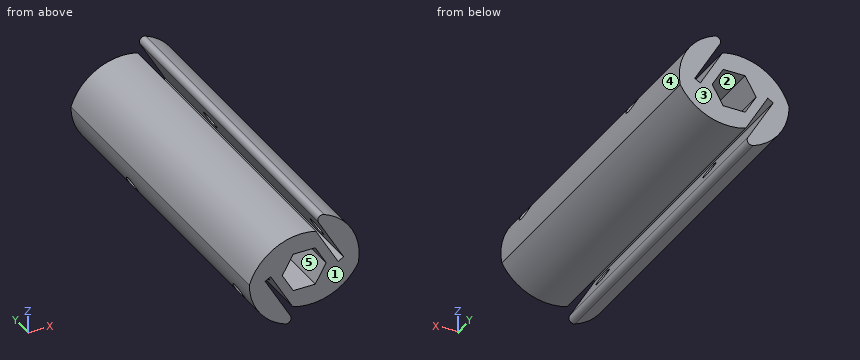
from build123d import *

# Parameters (mm, degrees)
BOSS_EXTRUDE1_DEPTH     = 114.3
CUT_EXTRUDE1_DEPTH      = 119.868393362
CUT_EXTRUDE1_DEPTH_BACK = 119.868393362
SKETCH2_R               = 3.175


with BuildPart() as part:
    # Sketch1 → Boss-Extrude1 (new body)
    with BuildSketch(Plane(origin=(0, 0, 0), x_dir=(1, 0, 0), z_dir=(0, 1, 0))):
        with BuildLine():
            Line((4.052973773, -12.538043503), (11.754987424, 0.80223546))
            Line((11.754987424, 0.80223546), (13.679728884, -0.30901454))
            Line((13.679728884, -0.30901454), (4.910037862, -15.498564956))
            ThreePointArc((4.910037862, -15.498564956), (5.078558502, -17.32430787), (6.856203481, -17.773434497))
            ThreePointArc((6.856203481, -17.773434497), (16.623747328, -9.303414683), (18.73470204, 3.451585069))
            ThreePointArc((18.73470204, 3.451585069), (8.97391608, 12.027162481), (-4.01489639, 12.349995465))
            Line((-4.01489639, 12.349995465), (-11.645002197, -0.86573546))
            Line((-11.645002197, -0.86573546), (-13.569743657, 0.24551454))
            Line((-13.569743657, 0.24551454), (-4.722290977, 15.569752099))
            ThreePointArc((-4.722290977, 15.569752099), (-4.884898453, 17.388542767), (-6.651388697, 17.851093199))
            ThreePointArc((-6.651388697, 17.851093199), (-15.646268799, 10.867233901), (-19.05, 0))
            ThreePointArc((-19.05, 0), (-10.00744853, -10.892061153), (4.052973773, -12.538043503))
        make_face()
        Polygon((3.812821178, -6.604), (7.625642355, 0), (3.812821178, 6.604), (-3.812821178, 6.604), (-7.625642355, 0), (-3.812821178, -6.604), align=None, mode=Mode.SUBTRACT)
    extrude(amount=BOSS_EXTRUDE1_DEPTH)

    # Sketch2 → Cut-Extrude1 (cut, two sides: drawn at the far end of the back side and taken through both)
    with BuildSketch(Plane(origin=(5.719231767, 0, 3.302), x_dir=(-0.5000000000000001, 0, 0.8660254037844386), z_dir=(-0.8660254037844386, 0, -0.5000000000000001)).offset(-CUT_EXTRUDE1_DEPTH_BACK)):
        with Locations(Location((0, 11.1125, 0), (0, 0, 180))):
            Circle(SKETCH2_R)
        with Locations(Location((0, 79.4385, 0), (0, 0, 180))):
            Circle(SKETCH2_R)
    extrude(amount=CUT_EXTRUDE1_DEPTH + CUT_EXTRUDE1_DEPTH_BACK, mode=Mode.SUBTRACT)


solid = part.part
For this review, take the finished solid that the model builds, in its own axes (mm). Face numbers are marked on the shaded views. A direction names the side the tool comes from. Give positions to 0.01 mm unless a question says otherwise; leave off trailing zeros.
Item 1: Draft analysis for pull direction X (two halves, no side actions). For the marked faces 3, 4 and 5, state which applies: +X half, -X half, draft (parallel to the pull), parting line (faces both ways), or undercut.
Item 2: Insertion check: pin 1 (2 mm diameter, centred on x = -7.5, y = 60, fed in from -Z); pin 2 (2 mm diameter, centred on x = 4, y = 66.5, fed in from -Z); pin 3 (5 mm diameter, centred on x = 2.5, y = 38.5, fed in from +Z). Each pin has a flat end and moves straight along its axis. Give the tip position at first contact, or say it passes through.
Item 3: For line 1 along X through (y, z) = (79, -5); line 2 along X through (y, z) = (47, -9); line 3 along Y through (x, z) = (8, 3.5), list the stretches that pass through material, from the lowest coordinate up.
Item 4: Take a section at B-B, the plane z = 4.5. Give the number of separate pieces and of enclosed holes in the cut face, and give its area (3 significant figures).
Item 5: Tool access review of the marked faces 1 and 2: name each direction out of +Z, -Z, +X, -X, +Y, -Y from which nothing blocks a thin tool from reaching the whole face with its end or side.
Calculated:
1. face 3: draft
1. face 4: +X half
1. face 5: undercut
2. pin 1: stops at z = -17.9
2. pin 2: stops at z = -13.31
2. pin 3: stops at z = 17.22
3. line 1: x = -18.38 to -14.95, 4.74 to 17.79
3. line 2: x = -16.79 to -8.52, -5.95 to 14.13
3. line 3: y = 0 to 8.09, 14.14 to 76.41, 82.46 to 114.3
4. separate pieces: 5
4. enclosed holes: 0
4. area: 2,540 mm2
5. face 1: +Z, -Z, +X, -X, -Y
5. face 2: +Y, -Y
